Here's how the part is built. I have some questions about the finished solid (model axes, mm). A direction names the side the tool comes from. Give positions to 0.01 mm unless a question says otherwise; leave off trailing zeros. Write each loop counter-clockwise with the first axis right and the second up, starting at its lowest first coordinate (ties: lowest second). Pieces come first, ordered by that corner, then holes. Notation, with made-up numbers: (-18.75, 70) - (-12.75, 70) arc R18 cw to (-12.75, 101) - close; hole circle Ø6 at (12.5, 55.25). An arc over 180 degrees is marked (long way). Use one line per item in the form item = value. Start each with the question number.
from build123d import *

# Parameters (mm, degrees)
SKETCH1_R                = 1.5
BOSS_EXTRUDE1_DEPTH      = 19
BOSS_EXTRUDE2_DEPTH      = 9.5
BOSS_EXTRUDE2_DEPTH_BACK = 9.5
SKETCH2_R                = 1.5
SKETCH3_R                = 1.5
SKETCH3_R_2              = 1.49
CUT_EXTRUDE1_DEPTH       = 3.5
CUT_EXTRUDE2_START       = -3.5
SKETCH4_R                = 1.5
SKETCH4_R_2              = 1.49
CUT_EXTRUDE2_DEPTH       = 3.5
CUT_EXTRUDE3_START       = -3.5
SKETCH5_R                = 1.5
SKETCH5_R_2              = 1.49
CUT_EXTRUDE3_DEPTH       = 3.5
SKETCH6_R                = 1.5
SKETCH6_R_2              = 1.49
CUT_EXTRUDE4_DEPTH       = 3.5


with BuildPart() as part:
    # Sketch1 → Boss-Extrude1 (new body)
    with BuildSketch(Plane(origin=(0, 0, 0), x_dir=(1, 0, 0), z_dir=(0, 1, 0))):
        with Locations(Location((0, 0, 0), (0, 0, 270))):
            Circle(SKETCH1_R)
    extrude(amount=BOSS_EXTRUDE1_DEPTH)

    # Sketch2 → Boss-Extrude2 (add, two sides: drawn at the far end of the back side and taken through both)
    with BuildSketch(Plane.XY.offset(-BOSS_EXTRUDE2_DEPTH_BACK)):
        with Locations((0, 9.5)):
            Circle(SKETCH2_R)
    extrude(amount=BOSS_EXTRUDE2_DEPTH + BOSS_EXTRUDE2_DEPTH_BACK)

    # Sketch3 → Cut-Extrude1 (cut)
    with BuildSketch(Plane(origin=(0, 0, -9.5), x_dir=(-1, 0, 0), z_dir=(0, 0, -1))):
        with Locations((0, 9.5)):
            Circle(SKETCH3_R)
        with Locations((0, 9.5)):
            Circle(SKETCH3_R_2, mode=Mode.SUBTRACT)
    extrude(amount=-CUT_EXTRUDE1_DEPTH, mode=Mode.SUBTRACT)

    # Sketch4 → Cut-Extrude2 (cut)
    with BuildSketch(Plane.XY.offset(9.5).offset(CUT_EXTRUDE2_START)):
        with Locations((0, 9.5)):
            Circle(SKETCH4_R)
        with Locations(Location((0, 9.5, 0), (0, 0, 180))):
            Circle(SKETCH4_R_2, mode=Mode.SUBTRACT)
    extrude(amount=CUT_EXTRUDE2_DEPTH, mode=Mode.SUBTRACT)

    # Sketch5 → Cut-Extrude3 (cut)
    with BuildSketch(Plane(origin=(0, 19, 0), x_dir=(1, 0, 0), z_dir=(0, 1, 0)).offset(CUT_EXTRUDE3_START)):
        with Locations(Location((0, 0, 0), (0, 0, 180))):
            Circle(SKETCH5_R)
        with Locations(Location((0, 0, 0), (0, 0, 270))):
            Circle(SKETCH5_R_2, mode=Mode.SUBTRACT)
    extrude(amount=CUT_EXTRUDE3_DEPTH, mode=Mode.SUBTRACT)

    # Sketch6 → Cut-Extrude4 (cut)
    with BuildSketch(Plane.XZ):
        with Locations(Location((0, 0, 0), (0, 0, 270))):
            Circle(SKETCH6_R)
        with Locations(Location((0, 0, 0), (0, 0, 90))):
            Circle(SKETCH6_R_2, mode=Mode.SUBTRACT)
    extrude(amount=-CUT_EXTRUDE4_DEPTH, mode=Mode.SUBTRACT)


solid = part.part
1. Please list where these lines run through material, in increasing order: line 1 (Y direction, x = 0.1, z = 3.25); line 2 (Z direction, x = 0.05, y = 14.25); line 3 (Y direction, x = -0.6, z = 3).
2. For P1, Ø2, axis at y = 7.5, z = 6, coming from the +X side, with a flat end and sliding along its axis, tell me the tip position at first contact or that it passes through.
3. I want a section at B-B, the plane y = 7. List the corners of the cut face in (x, z) for me.
4. For faces 1 (the face through (-1.5, 9.57, -3.71)), 2 (the face through (-1.477, 1.726, -0.194)), 3 (the face through (0.323, 10.955, 7.726)), 4 (the face through (1.477, 17.226, -0.194)), which set-ups out of +Z, -Z, +X, -X, +Y, -Y let a thin tool reach every point of the face, with its end or its side?
5. I want a section at C-C, the plane z = -6.5. List the corners of the cut face in (x, y) for me.
Result sheet:
q1.line_1 = 8 to 11
q1.line_2 = -1.5 to 1.5
q1.line_3 = 8.13 to 10.87
q2.P1 = 1.12
q3.outline = circle Ø3 at (0, 0)
q4.face_1 = -Z
q4.face_2 = -Y
q4.face_3 = +Z
q4.face_4 = +Y
q5.outline = circle Ø2.98 at (0, 9.5)
